```python
from build123d import *

# Parameters (mm, degrees)
SKETCH1_R           = 4
SKETCH1_R_2         = 2.3
BOSS_EXTRUDE1_DEPTH = 3.2
SKETCH2_R           = 4
SKETCH2_R_2         = 0.85
BOSS_EXTRUDE2_DEPTH = 2
BOSS_EXTRUDE3_DEPTH = 8
SKETCH6_R           = 0.85
CUT_EXTRUDE1_DEPTH  = 2


with BuildPart() as part:
    # Sketch1 → Boss-Extrude1 (new body)
    with BuildSketch(Plane.XY):
        Circle(SKETCH1_R)
        Circle(SKETCH1_R_2, mode=Mode.SUBTRACT)
    extrude(amount=-BOSS_EXTRUDE1_DEPTH)

    # Sketch2 → Boss-Extrude2 (add)
    with BuildSketch(Plane.XY):
        Circle(SKETCH2_R)
        Circle(SKETCH2_R_2, mode=Mode.SUBTRACT)
    extrude(amount=BOSS_EXTRUDE2_DEPTH)

    # Sketch5 → Boss-Extrude3 (add)
    with BuildSketch(Plane(origin=(3.819651946, -1.187543266, 0), x_dir=(0, 0, -1), z_dir=(0.954912987, -0.296885816, 0))):
        Polygon((-2, 0), (3.2, 0), (3.2, -17.878888538), (-2, -17.878888538), (-2, -17.94433562), (-22.731913212, -17.94433562), (-22.731913212, -9.94433562), (-2, -9.94433562), align=None)
    extrude(amount=-BOSS_EXTRUDE3_DEPTH)

    # Sketch6 → Cut-Extrude1 (cut)
    with BuildSketch(Plane.XY.offset(2)):
        Circle(SKETCH6_R)
    extrude(amount=-CUT_EXTRUDE1_DEPTH, mode=Mode.SUBTRACT)


solid = part.part
```
Design review of the part built by this model. Coordinates are the model's own, in mm. A direction names the side the tool comes from. Give positions to 0.01 mm unless a question says otherwise; leave off trailing zeros. Write each loop counter-clockwise with the first axis right and the second up, starting at its lowest first coordinate (ties: lowest second). Pieces come first, ordered by that corner, then holes.
(1) Tool access review of faces 1 (the face through (-2.899, -9.513, 12.511)), 2 (the face through (-5.25, -17.09, -0.64)), 3 (the face through (0, -0.3, 0)), 4 (the face through (0, 0, -2)): name each direction out of +Z, -Z, +X, -X, +Y, -Y from which nothing blocks a thin tool from reaching the whole face with its end or side.
Checked values:
face 1: +Z, +X, +Y
face 2: -Z, -X, -Y
face 3: +Z
face 4: -Z
(2) Wall thickness on line 1 along Z through (x, y) = (1, 2); line 2 along Z through (x, y) = (0.25, -2.5); line 3 along X through (y, z) = (0, 1): over which ranges is each line inside the solid? List them lowest first.
Checked values:
line 1: z = 0 to 2
line 2: z = -3.2 to 2
line 3: x = -4.19 to -0.85, 0.85 to 4
(3) Add section C-C (z = 6). Give the boundary of the cut face in (x, y).
Checked values:
outline: (-9.15, -15.95) - (-1.51, -18.32) - (0.87, -10.68) - (-6.77, -8.31) - close
(4) Add section D-D (y = -9). Give the boundary of the cut face in (x, z).
Checked values:
outline: (-6.99, -3.2) - (1.39, -3.2) - (1.39, 2) - (-4.55, 2) - (-4.55, 22.73) - (-6.99, 22.73) - close
(5) Add section B-B (x = -0.5). Give the boundary of the cut face in (y, z) (3 decimals).
Checked values:
outline: (-15.081, -3.2) - (0.155, -3.2) - (0.155, 0) - (-0.687, 0) - (-0.687, 2) - (-10.258, 2) - (-10.258, 22.732) - (-15.081, 22.732) - close; (0.687, 0) - (2.245, 0) - (2.245, -3.2) - (3.969, -3.2) - (3.969, 2) - (0.687, 2) - close
(6) Add section A-A (z = -0.75). Give the boundary of the cut face in (x, y), and give its area (3 significant figures).
Checked values:
outline: (-9.13, -15.89) - (-1.49, -18.26) - (3.82, -1.19) arc R4 ccw to (-3.82, 1.19) - close; hole (-2.2, 0.68) - (2.2, -0.68) arc R2.3 ccw to start
area: 160 mm2
(7) Clearance check with flat-ended pins moving along their axes: pin 1 Ø1 at (y, z) = (-11.5, 3.5) entering from +X; pin 2 Ø1.5 at (x, y) = (-0.5, -5) entering from +Z; pin 3 Ø6 at (y, z) = (-9.5, 16) entering from +X. State where each tip first meets the part, or that it passes through.
Checked values:
pin 1: stops at x = 0.77
pin 2: stops at z = 2
pin 3: stops at x = 0.87
(8) Mouldability with a two-part tool opening along X and no side actions: class faces 5 (the face through (-0.653, 0.544, 0.986)), 6 (the face through (0.01, -13.44, 6.7)), 7 (the face through (-7.63, -11.07, 6.7)) as +X half, -X half, draft (parallel to the pull), parting line (faces both ways), or undercut.
Checked values:
face 5: undercut
face 6: +X half
face 7: -X half
